from build123d import *

# Parameters (mm, degrees)
EXTRUDE_1_DEPTH     = 20
SKETCH_3_R          = 4
CUT_EXTRUDE_1_DEPTH = 20


with BuildPart() as part:
    # 草图1 → 凸台-拉伸1 (new body)
    with BuildSketch(Plane(origin=(0, 0, 0), x_dir=(0, 0, -1), z_dir=(1, 0, 0))):
        with BuildLine():
            Line((-15, 24), (1.928932188, 7.071067812))
            ThreePointArc((1.928932188, 7.071067812), (4.857864376, 0), (1.928932188, -7.071067812))
            Line((1.928932188, -7.071067812), (-15, -24))
            Line((-15, -24), (-15, -42.5))
            Line((-15, -42.5), (15, -42.5))
            Line((15, -42.5), (15, 42.5))
            Line((15, 42.5), (-15, 42.5))
            Line((-15, 42.5), (-15, 24))
        make_face()
    extrude(amount=EXTRUDE_1_DEPTH)

    # 草图3 → 切除-拉伸1 (cut)
    with BuildSketch(Plane.ZY):
        with Locations((0, 26.25)):
            Circle(SKETCH_3_R)
        with Locations(Location((0, -26.25, 0), (0, 0, 180))):
            Circle(SKETCH_3_R)
    extrude(amount=-CUT_EXTRUDE_1_DEPTH, mode=Mode.SUBTRACT)


solid = part.part
The listing builds one solid part. Answer for the finished solid, in the listing's coordinates (mm). A direction names the side the tool comes from. Give positions to 0.01 mm unless a question says otherwise; leave off trailing zeros. Loops run counter-clockwise (first coordinate to the right, second up) from the corner with the lowest first, then second, coordinate; pieces in that order, holes last. Notation, with made-up numbers: M -32,-37.5 L -26,-37.5 A24 cw -26,-24.5 Z; hole C 15,10 d2. An arc over 180 degrees is marked long. Answer as CSV lines item,"result".
Item 1: The mould has two halves that part along Y. Classify faces 3 (the flat face through (10, 16, 7)), 4 (the cylindrical face through (9.86, 30.216, -0.521)), 5 (the flat face through (10, 42.5, 0)), 6 (the flat face through (20, 1, -6)): released by +Y, released by -Y, zero draft, split by the parting line, or undercut.
Values follow:
face 3,"undercut"
face 4,"undercut"
face 5,"released by +Y"
face 6,"zero draft"
Item 2: Which of the six approach directions +Z, -Z, +X, -X, +Y, -Y give full straight-line access (tool end or side, diameter ignored) to faces 1 (the flat face through (10, 33, 15)), 2 (the flat face through (10, -15, 6))?
Values follow:
face 1,"+Z, +X, -X, +Y, -Y"
face 2,"+Z, +X, -X"
Item 3: Given pin 1 Ø8 at (x, y) = (10, 15.5) entering from +Z, flat-ended and moving along its own axis, determine where the tip first touches the part or whether it passes through.
Values follow:
pin 1,"stops at z = 10.5"
Item 4: The part is cut by section A-A (z = 0). Give the vertices of the cut face in (x, y).
Values follow:
outline,"M 0,-42.5 L 20,-42.5 L 20,-30.25 L 0,-30.25 Z; M 0,-22.25 L 20,-22.25 L 20,-9 L 0,-9 Z; M 0,9 L 20,9 L 20,22.25 L 0,22.25 Z; M 0,30.25 L 20,30.25 L 20,42.5 L 0,42.5 Z"
Item 5: The part is cut by section B-B (y = 26.25). Give the vertices of the cut face in (x, z).
Values follow:
outline,"M 0,-15 L 20,-15 L 20,-4 L 0,-4 Z; M 0,4 L 20,4 L 20,15 L 0,15 Z"
Item 6: Straight lines are drawn through the part: line 1 along Y through (x, z) = (8.75, 0); line 2 along Z through (x, y) = (9.75, -26.25); line 3 along Y through (x, z) = (10.75, -0.25). For each, find the intervals that lie inside material, in ascending order. Write a range as [from, to].
Values follow:
line 1,"y = [-42.5, -30.25], [-22.25, -9], [9, 22.25], [30.25, 42.5]"
line 2,"z = [-15, -4], [4, 15]"
line 3,"y = [-42.5, -30.24], [-22.26, -8.75], [8.75, 22.26], [30.24, 42.5]"
Item 7: The part is cut by section C-C (z = 10.5). Give the vertices of the cut face in (x, y).
Values follow:
outline,"M 0,-42.5 L 20,-42.5 L 20,-19.5 L 0,-19.5 Z; M 0,19.5 L 20,19.5 L 20,42.5 L 0,42.5 Z"
Item 8: The part is cut by section D-D (x = 8). Give the vertices of the cut face in (y, z), and give its area (3 significant figures).
Values follow:
outline,"M -42.5,-15 L 42.5,-15 L 42.5,15 L 24,15 L 7.07,-1.93 A10 cw -7.07,-1.93 L -24,15 L -42.5,15 Z; hole C -26.25,0 d8; hole C 26.25,0 d8"
area,"1,890 mm^2"
